Build history of the part. All positions in model axes, mm. Round coordinates to 2 decimals unless told otherwise and drop trailing zeros. Write each loop counter-clockwise with the first axis right and the second up, starting at its lowest first coordinate (ties: lowest second). Pieces come first, ordered by that corner, then holes.
Item 1: Band-saw the part on B-B, the plane z = 2.05. Count the separate pieces of the cut face and the enclosed holes in it, then the cut area to 3 significant figures.
Item 2: Band-saw the part on A-A, the plane x = -61. Write the cut outline in (y, z), then the cut area to 3 significant figures.
Item 3: Band-saw the part on D-D, the plane x = 52. Write the cut outline in (y, z), then the cut area to 3 significant figures.
Item 4: Wall check: probe 1 along Y at (x, z) = (17.5, 2.1); probe 2 along Y at (x, z) = (53, 0.3); probe 3 along Y at (x, z) = (17, 0.6). Give the ranges that are in metal, low to high.
Item 5: Drop flat-ended pins along their axis: pin 1 Ø2 at (x, z) = (63.5, 2) entering from +Y; pin 2 Ø2 at (y, z) = (135, 3) entering from +X; pin 3 Ø1.5 at (x, z) = (13, 3.5) entering from -Y. Give the stop position or say it passes through.
Item 6: Band-saw the part on C-C, the plane y = 155. Write the cut outline in (x, z), then the cut area to 3 significant figures.
```python
from build123d import *

# Parameters (mm, degrees)
F0_R     = 1.75
F0_R_2   = 4
F0_R_3   = 2.5
F0_R_4   = 2.25
F1_DEPTH = 4


with BuildPart() as f1:
    # F0 (on Top) → F1 (new body)
    with BuildSketch(Plane.XY):
        with BuildLine():
            ThreePointArc((80, 169.488149), (0, 219.488149), (-80, 169.488149))
            Line((-80, 169.488149), (-40, 169.488149))
            Line((-40, 169.488149), (-40, 99.488149))
            Line((-40, 99.488149), (-80, 99.488149))
            Line((-80, 99.488149), (-80, -22.511851))
            Line((-80, -22.511851), (-40, -22.511851))
            Line((-40, -22.511851), (-40, -92.511851))
            Line((-40, -92.511851), (-80, -92.511851))
            ThreePointArc((-80, -92.511851), (0, -142.511851), (80, -92.511851))
            Line((80, -92.511851), (40, -92.511851))
            Line((40, -92.511851), (40, -22.511851))
            Line((40, -22.511851), (80, -22.511851))
            Line((80, -22.511851), (80, 99.488149))
            Line((80, 99.488149), (40, 99.488149))
            Line((40, 99.488149), (40, 169.488149))
            Line((40, 169.488149), (80, 169.488149))
        make_face()
        with Locations((-44, -1.511851)):
            Circle(F0_R, mode=Mode.SUBTRACT)
        with Locations((-17.5, -38.761851)):
            Circle(F0_R, mode=Mode.SUBTRACT)
        with Locations((-20, -26.511851)):
            Circle(F0_R_2, mode=Mode.SUBTRACT)
        with Locations((-18, 19.488149)):
            Circle(F0_R_3, mode=Mode.SUBTRACT)
        with Locations((17.5, -38.761851)):
            Circle(F0_R, mode=Mode.SUBTRACT)
        with Locations((20, -26.511851)):
            Circle(F0_R_2, mode=Mode.SUBTRACT)
        with Locations((25, -16.511851)):
            Circle(F0_R_3, mode=Mode.SUBTRACT)
        with Locations((44, -1.511851)):
            Circle(F0_R, mode=Mode.SUBTRACT)
        with Locations((-44, 38.488149)):
            Circle(F0_R, mode=Mode.SUBTRACT)
        with Locations((-44, 78.488149)):
            Circle(F0_R, mode=Mode.SUBTRACT)
        with Locations((-18, 58.488149)):
            Circle(F0_R_3, mode=Mode.SUBTRACT)
        with Locations((-20, 109.488149)):
            Circle(F0_R_2, mode=Mode.SUBTRACT)
        with Locations((25, 93.488149)):
            Circle(F0_R_3, mode=Mode.SUBTRACT)
        with Locations((20, 109.488149)):
            Circle(F0_R_2, mode=Mode.SUBTRACT)
        with Locations((44, 38.488149)):
            Circle(F0_R, mode=Mode.SUBTRACT)
        with Locations((44, 78.488149)):
            Circle(F0_R, mode=Mode.SUBTRACT)
        with Locations((0, 140.488149)):
            Circle(F0_R_4, mode=Mode.SUBTRACT)
        with Locations((0, 215.488149)):
            Circle(F0_R, mode=Mode.SUBTRACT)
    extrude(amount=F1_DEPTH)


solid = f1.part
```
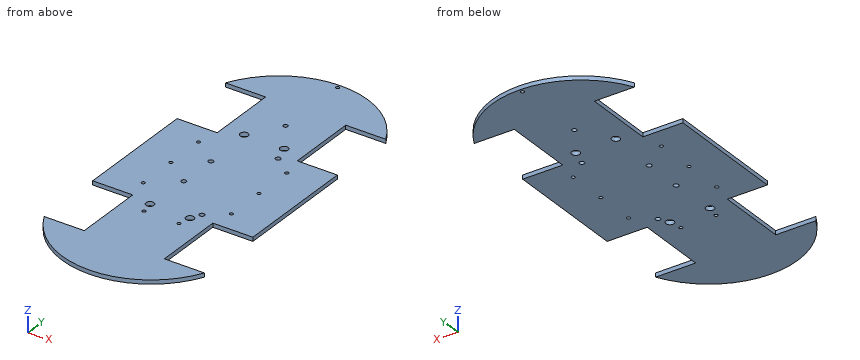
Results:
1. separate pieces: 1
1. enclosed holes: 18
1. area: 41,800 mm2
2. outline: (-118.32, 0) - (-92.51, 0) - (-92.51, 4) - (-118.32, 4) - close; (-22.51, 0) - (99.49, 0) - (99.49, 4) - (-22.51, 4) - close; (169.49, 0) - (195.3, 0) - (195.3, 4) - (169.49, 4) - close
2. area: 694 mm2
3. outline: (-125.74, 0) - (-92.51, 0) - (-92.51, 4) - (-125.74, 4) - close; (-22.51, 0) - (99.49, 0) - (99.49, 4) - (-22.51, 4) - close; (169.49, 0) - (202.72, 0) - (202.72, 4) - (169.49, 4) - close
3. area: 754 mm2
4. probe 1: y = -140.77 to -40.51, -37.01 to -29.63, -23.39 to 106.37, 112.61 to 217.75
4. probe 2: y = -125.01 to -92.51, -22.51 to 99.49, 169.49 to 201.99
4. probe 3: y = -140.87 to -40.44, -37.08 to -29.16, -23.87 to 106.84, 112.13 to 217.85
5. pin 1: stops at y = 193.85
5. pin 2: stops at x = 40
5. pin 3: stops at y = -141.66
6. outline: (-40, 0) - (40, 0) - (40, 4) - (-40, 4) - close
6. area: 320 mm2
